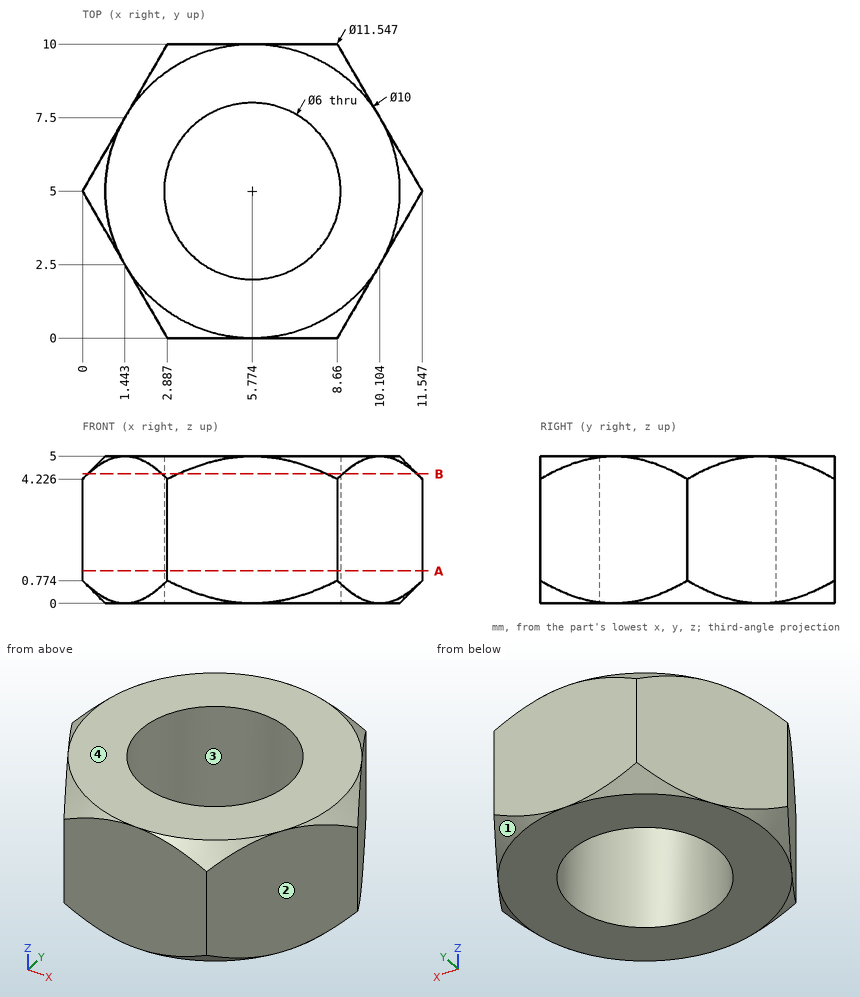
Answer from the drawing. Dimensions are ordinates in mm from the lowest x, y and z of the part. Give positions to 0.01 mm unless a question says otherwise; leave off trailing zeros. Loops run counter-clockwise (first coordinate to the right, second up) from the corner with the lowest first, then second, coordinate; pieces in that order, holes last. Notation, with made-up numbers: M 58,-20 L 116,-20 A28 ccw 116,7 Z; hole C -2.75,12 d8. An arc over 180 degrees is marked long. One line per item, written item: value.
Q1. Flat-ended cylindrical pins translate along their axes: P1, Ø2, axis at x = 10, z = 1.5, coming from the +Y side; P2, Ø2, axis at x = 4, z = 2, coming from the -Y side; P3, Ø1.5, axis at y = 2, z = 3.5, coming from the -X side; P4, Ø3.5, axis at x = 5.77, y = 5, coming from the -Z side. Find the tip coordinate at first contact, or state that the pin passes through.
Working result:
P1: stops at y = 9.41
P2: stops at y = 0
P3: stops at x = 1.3
P4: passes through
Q2. Find the intervals of material crossed by line 1 (X direction, y = 3, z = 1.4) (1 decimal); line 2 (X direction, y = 6, z = 1.1) (1 decimal); line 3 (Y direction, x = 3.5, z = 1.5) (1 decimal), in increasing order. Write a range as from..to.
Working result:
line 1: x = 1.2..3.5, 8..10.4
line 2: x = 0.6..2.9, 8.6..11
line 3: y = 0..3, 7..10
Q3. Determine the mould class of the marked faces 1, 2, 3 and 4 for opening direction Y: +Y half, -Y half, draft (parallel to the pull), parting line (faces both ways), or undercut.
Working result:
face 1: +Y half
face 2: -Y half
face 3: undercut
face 4: draft
Q4. A cutting plane is placed at A-A on z = 1.1. Determine the outline of the cut face in (x, y).
Working result:
outline: M 0,5 L 2.89,0 L 8.66,0 L 11.55,5 L 8.66,10 L 2.89,10 Z; hole C 5.77,5 d6
Q5. A cutting plane is placed at B-B on z = 4.4. Determine the outline of the cut face in (x, y) (1 decimal).
Working result:
outline: M 0.2,4.7 L 2.7,0.3 A5.6 ccw 3.3,0 L 8.3,0 A5.6 ccw 8.8,0.3 L 11.4,4.7 A5.6 ccw 11.4,5.3 L 8.8,9.7 A5.6 ccw 8.3,10 L 3.3,10 A5.6 ccw 2.7,9.7 L 0.2,5.3 A5.6 ccw Z; hole C 5.8,5 d6
